CAD build for the part. Positions are in the model's coordinates, mm. A direction names the side the tool comes from. Coordinates: 2 decimals unless noted, no trailing zeros. Loops run counter-clockwise (first coordinate to the right, second up) from the corner with the lowest first, then second, coordinate; pieces in that order, holes last. Notation, with made-up numbers: (77.25, 57) - (97.25, 57) arc R22 cw to (97.25, 96) - close; hole circle Ø9 at (42, 34.5). An arc over 180 degrees is marked (long way). Put each result on its own line as item: value.
```python
from build123d import *

# Parameters (mm, degrees)
F0_W     = 144.1599577665
F0_H     = 87.3491168022
F1_DEPTH = 25.4
F2_T     = -2.54
F3_R     = 7.7655304072
F4_DEPTH = 25.4


with BuildPart() as f1:
    # F0 (on Top) → F1 (new body)
    with BuildSketch(Plane.XY):
        with Locations((9.7206383944, -22.1865028143)):
            Rectangle(F0_W, F0_H)
    extrude(amount=F1_DEPTH)

    # F2
    f2_openings = [f1.faces().sort_by_distance(p)[0] for p in [
        (9.720638, -22.186503, 25.4),
    ]]
    offset(amount=F2_T, openings=f2_openings)

    # F3 (on face) → F4 (join)
    with BuildSketch(Plane.XZ.offset(65.8610612154)):
        with Locations((-46.0575036705, 11.1663378775)):
            Circle(F3_R)
    extrude(amount=F4_DEPTH)


solid = f1.part
```
Q1. Slice it at C-C, the plane x = 63.5. Give the cut face in (y, z).
Determined:
outline: (-65.86, 0) - (21.49, 0) - (21.49, 25.4) - (18.95, 25.4) - (18.95, 2.54) - (-63.32, 2.54) - (-63.32, 25.4) - (-65.86, 25.4) - close
Q2. Slice it at A-A, the plane z = 23.25. Give the cut face in (x, y).
Determined:
outline: (-62.36, -65.86) - (81.8, -65.86) - (81.8, 21.49) - (-62.36, 21.49) - close; hole (-59.82, -63.32) - (79.26, -63.32) - (79.26, 18.95) - (-59.82, 18.95) - close
Q3. Slice it at D-D, the plane z = 13. Give the cut face in (x, y), then the cut area to 3 significant figures.
Determined:
outline: (-62.36, -65.86) - (-53.6, -65.86) - (-53.6, -91.26) - (-38.51, -91.26) - (-38.51, -65.86) - (81.8, -65.86) - (81.8, 21.49) - (-62.36, 21.49) - close; hole (-59.82, -63.32) - (79.26, -63.32) - (79.26, 18.95) - (-59.82, 18.95) - close
area: 1,530 mm2
Q4. Wall check: L1, parallel to Y at x = -5.5, z = 14.5; L2, parallel to X at y = -46, z = 4.5; L3, parallel to Y at x = -47.5, z = 15.5. Give the ranges that are in metal, low to high. Write a range as from..to.
Determined:
L1: -65.86..-63.32, 18.95..21.49
L2: -62.36..-59.82, 79.26..81.8
L3: -91.26..-63.32, 18.95..21.49
Q5. Slice it at B-B, the plane y = -35. Give the cut face in (x, z).
Determined:
outline: (-62.36, 0) - (81.8, 0) - (81.8, 25.4) - (79.26, 25.4) - (79.26, 2.54) - (-59.82, 2.54) - (-59.82, 25.4) - (-62.36, 25.4) - close
Q6. Pin check, flat tips, straight feed: pin 1 Ø6 at (y, z) = (-69, 11.5) entering from -X; pin 2 Ø1.5 at (x, y) = (7, -40.5) entering from -Z; pin 3 Ø8 at (x, z) = (4.5, 6.5) entering from -Y. Stop position of each tip, or through.
Determined:
pin 1: x = -53.82
pin 2: z = 0
pin 3: y = -65.86
Q7. Mould opens along Y. For faces 1 (the cylindrical face through (-53.816, -78.383, 11.508)), 2 (the flat face through (9, -22, 2.54)), 3 (the flat face through (9, 21.488, 13)), 4 (the flat face through (79.261, -23, 14)) say: +Y half, -Y half, draft (parallel to the pull), parting line (faces both ways), or undercut.
Determined:
face 1: draft
face 2: undercut
face 3: +Y half
face 4: undercut
Q8. Tool access for faces 5 (the flat face through (9, 18.948, 14)), 6 (the flat face through (81.801, -23, 13)): list every direction of +Z, -Z, +X, -X, +Y, -Y with a clear straight run to the whole face (end or side of a thin tool).
Determined:
face 5: +Z
face 6: +Z, -Z, +X, +Y, -Y
